```python
from build123d import *

# Parameters (mm, degrees)
SKETCH1_R           = 7
SKETCH1_R_2         = 3
BOSS_EXTRUDE1_DEPTH = 6
SKETCH2_R           = 4
SKETCH2_R_2         = 3
BOSS_EXTRUDE2_DEPTH = 0.5
FILLET1_R           = 0.3
FILLET2_R           = 0.25
CIRPATTERN1_COUNT   = 2
CIRPATTERN1_ANGLE   = 90


# Read off the part's stored shape, not the designer's step: M4 Tapped Hole1
with BuildPart() as part:
    # Sketch1 → Boss-Extrude1 (new body)
    with BuildSketch(Plane(origin=(0, 0, 0), x_dir=(1, 0, 0), z_dir=(0, 1, 0))):
        with Locations(Location((0, 0, 0), (0, 0, 270))):
            Circle(SKETCH1_R)
        with Locations(Location((0, 0, 0), (0, 0, 270))):
            Circle(SKETCH1_R_2, mode=Mode.SUBTRACT)
    extrude(amount=BOSS_EXTRUDE1_DEPTH)

    # Sketch2 → Boss-Extrude2 (add)
    with BuildSketch(Plane(origin=(0, 6, 0), x_dir=(1, 0, 0), z_dir=(0, 1, 0))):
        with Locations(Location((0, 0, 0), (0, 0, 270))):
            Circle(SKETCH2_R)
        with Locations(Location((0, 0, 0), (0, 0, 270))):
            Circle(SKETCH2_R_2, mode=Mode.SUBTRACT)
    extrude(amount=BOSS_EXTRUDE2_DEPTH)

    # Fillet1
    fillet1_edges = [part.edges().sort_by_distance(p)[0] for p in [
        (0, 6.5, -4),
        (0, 6.5, -3),
    ]]
    fillet(fillet1_edges, radius=FILLET1_R)

    # Fillet2
    fillet2_edges = [part.edges().sort_by_distance(p)[0] for p in [
        (0, 0, -7),
        (0, 6, -7),
    ]]
    fillet(fillet2_edges, radius=FILLET2_R)

    # M4 Tapped Hole1 outline → M4 Tapped Hole1 (revolve, cut)
    with BuildSketch(Plane.XZ.offset(-3)):
        Polygon((2.025001015, 7.000001015), (0, 7.000001015), (0, 2.505277626), (1.65, 2.505277626), (1.65, 6.625), align=None)
    m4_tapped_hole1 = revolve(axis=Axis((0, 3, 0), (0, 0, 1)), mode=Mode.SUBTRACT)

    # CirPattern1: M4 Tapped Hole1 ×2 about axis
    cirpattern1_axis = Axis((0, 6, 0), (0, -1, 0))
    for i in range(1, CIRPATTERN1_COUNT):
        add(m4_tapped_hole1.rotate(cirpattern1_axis, i * CIRPATTERN1_ANGLE / (CIRPATTERN1_COUNT - 1)), mode=Mode.SUBTRACT)


solid = part.part
```
Verification items for the finished model (mm, model axes). A direction names the side the tool comes from. Give positions to 0.01 mm unless a question says otherwise; leave off trailing zeros. Loops run counter-clockwise (first coordinate to the right, second up) from the corner with the lowest first, then second, coordinate; pieces in that order, holes last.
1. Section check A-A, the plane x = 0. Enter the section's corners in (y, z) (3 decimals).
2. Section check B-B, the plane z = 0. Enter the section's corners in (x, y) (3 decimals), then the cut area to 3 significant figures.
3. Go/stop test with flat-tipped pins: pin 1 Ø4 at (x, z) = (-5.5, -4) entering from +Y; pin 2 Ø3 at (x, y) = (0, 3) entering from +Z; pin 3 Ø3 at (x, z) = (4, 3.5) entering from +Y. Record where each tip stops, or that it passes through.
4. Set-up check for faces 4 (the cylindrical face through (-4.59, 3.07, -1.65)), 5 (the flat face through (-3, 6, 3)), 6 (the flat face through (-1, 0, 3)): record each of +Z, -Z, +X, -X, +Y, -Y from which the full face is reachable in a straight line by a thin tool's end or side.
5. Section check C-C, the plane y = 5.5. Enter the section's corners in (x, z).
6. Mould release check, pull along Z, two halves, no side actions. Record for faces 1 (the cylindrical face through (5.902, 2.962, 3.763)), 2 (the cylindrical face through (-1.65, 3.07, 4.59)), 3 (the cylindrical face through (2.03, 3.06, -2.21)): released by +Z, released by -Z, zero draft, split by the parting line, or undercut.
7. Thickness scan on line 1 (Y direction, x = -3.25, z = 0); line 2 (Y direction, x = -1.25, z = -4); line 3 (X direction, y = 2, z = 2.5). Record the ranges inside material, lowest first.
Geometry says:
1. outline: (0, -6.75) arc R0.25 ccw to (0.25, -7) - (5.75, -7) arc R0.25 ccw to (6, -6.75) - (6, -4) - (6.2, -4) arc R0.3 ccw to (6.5, -3.7) - (6.5, -3.3) arc R0.3 ccw to (6.2, -3) - (0, -3) - close; (0, 3) - (1.35, 3) - (1.35, 6.625) - (0.975, 7) - (0.25, 7) arc R0.25 ccw to (0, 6.75) - close; (4.65, 3) - (6.2, 3) arc R0.3 ccw to (6.5, 3.3) - (6.5, 3.7) arc R0.3 ccw to (6.2, 4) - (6, 4) - (6, 6.75) arc R0.25 ccw to (5.75, 7) - (5.025, 7) - (4.65, 6.625) - close
2. outline: (-7, 0.25) arc R0.25 ccw to (-6.75, 0) - (-3, 0) - (-3, 1.35) - (-6.625, 1.35) - (-7, 0.975) - close; (-7, 5.025) - (-6.625, 4.65) - (-3, 4.65) - (-3, 6.2) arc R0.3 ccw to (-3.3, 6.5) - (-3.7, 6.5) arc R0.3 ccw to (-4, 6.2) - (-4, 6) - (-6.75, 6) arc R0.25 ccw to (-7, 5.75) - close; (3, 0) - (6.75, 0) arc R0.25 ccw to (7, 0.25) - (7, 5.75) arc R0.25 ccw to (6.75, 6) - (4, 6) - (4, 6.2) arc R0.3 ccw to (3.7, 6.5) - (3.3, 6.5) arc R0.3 ccw to (3, 6.2) - close
2. area: 35.5 mm2
3. pin 1: stops at y = 6
3. pin 2: stops at z = -2.6
3. pin 3: stops at y = 6.48
4. face 4: -X
4. face 5: +Y
4. face 6: +Z, -Z, +X, -X, -Y
5. outline: circle Ø14 at (0, 0); hole circle Ø6 at (0, 0)
6. face 1: split by the parting line
6. face 2: zero draft
6. face 3: undercut
7. line 1: y = 0 to 1.35, 4.65 to 6.5
7. line 2: y = 0 to 6
7. line 3: x = -6.54 to -1.66, 1.66 to 6.54
